CAD build for the part. Positions are in the model's coordinates, mm. Coordinates: 2 decimals unless noted, no trailing zeros. Loops run counter-clockwise (first coordinate to the right, second up) from the corner with the lowest first, then second, coordinate; pieces in that order, holes last.
1) Pin check, flat tips, straight feed: pin 1 Ø8 at (x, y) = (-15.5, 11) entering from -Z; pin 2 Ø10 at (y, z) = (25.5, 25.5) entering from +X; pin 3 Ø4 at (x, z) = (25, 29) entering from -Y. Stop position of each tip, or through.
2) Saw through at C-C, the plane z = 49.5. Write the cut outline in (x, y).
3) Wall check: line 1 along Y through (x, z) = (0, -0.4); line 2 along X through (y, z) = (-7, 47); line 3 along X through (y, z) = (69, 16.5). Give the ranges that are in metal, low to high.
4) Two-plate mould, pull along Y, no slides. Class faces 1 (the cylindrical face through (80.422, 3.539, -0.986)), 2 (the flat face through (-59, -53, 0)), 3 (the cylindrical face through (16.66, -75.023, -0.986)): +Y half, -Y half, draft (parallel to the pull), parting line (faces both ways), or undercut.
5) Saw through at A-A, the plane x = 0. Write the cut outline in (y, z), and give its area (3 significant figures).
```python
from build123d import *

# Parameters (mm, degrees)
SHELL1_T            = -2
SKETCH2_R           = 80.5
SKETCH2_R_2         = 76.85
BOSS_EXTRUDE1_DEPTH = 2


# Read off the part's stored shape, not the designer's step: Revolve1
with BuildPart() as part:
    # Revolve1 outline → Revolve1 (revolve)
    with BuildSketch(Plane.XZ):
        with BuildLine():
            Line((0, 0), (78.85, -7.9e-08))
            ThreePointArc((78.85, -7.9e-08), (55.755369724, 55.755369669), (0, 78.85))
            Line((0, 78.85), (0, 0))
        make_face()
    revolve(axis=Axis((0, 0, 0), (0, 0, 1)))

    # Shell1
    shell1_openings = [part.faces().sort_by_distance(p)[0] for p in [
        (0, 0, 0),
    ]]
    offset(amount=SHELL1_T, openings=shell1_openings, kind=Kind.INTERSECTION)

    # Sketch2 → Boss-Extrude1 (add)
    with BuildSketch(Plane(origin=(0, 0, 0), x_dir=(-1, 0, 0), z_dir=(0, 0, -1))):
        Circle(SKETCH2_R)
        Circle(SKETCH2_R_2, mode=Mode.SUBTRACT)
    extrude(amount=BOSS_EXTRUDE1_DEPTH)


solid = part.part
```
Data:
1. pin 1: stops at z = 73.33
1. pin 2: stops at x = 72.47
1. pin 3: stops at y = -70
2. outline: circle Ø122.75 at (0, 0); hole circle Ø117.57 at (0, 0)
3. line 1: y = -80.5 to -76.85, 76.85 to 80.5
3. line 2: x = -62.92 to -60.4, 60.4 to 62.92
3. line 3: x = -34.41 to -29.54, 29.54 to 34.41
4. face 1: parting line
4. face 2: draft
4. face 3: undercut
5. outline: (-80.5, -2) - (-76.85, -2) - (-76.85, 0) arc R76.85 cw to (76.85, 0) - (76.85, -2) - (80.5, -2) - (80.5, 0) - (78.85, 0) arc R78.85 ccw to (-78.85, 0) - (-80.5, 0) - close
5. area: 504 mm2
